Autodesk Inventor part; units mm, degrees
ref_plane "YZ Plane" through (0, 0, 0) normal (1, 0, 0) x (0, 1, 0)
ref_plane "XZ Plane" through (0, 0, 0) normal (0, 1, 0) x (-1, 0, 0)
ref_plane "XY Plane" through (0, 0, 0) normal (0, 0, 1) x (1, 0, 0)
sketch "スケッチ1" plane through (0, 0, 0) normal (0, 0, 1) x (1, 0, 0)
  circle A0 centre (0, 0) radius 2.5
  dimension "d0" = 5
extrude "押し出し1" add sketch "スケッチ1" along normal blind 7.7
fillet "フィレット1" radius 2.5 1 edges at (-2.5, 0, 7.7)
sketch "スケッチ2" plane through (0, 0, 0) normal (0, 0, -1) x (-1, 0, 0)
  circle A0 centre (0, 0) radius 2.9
  line L0 (2.5, 1.4697) -> (2.5, -1.4697)
  circle A1 centre (0, 0) radius 2.5
  dimension "d4" = 5.8
extrude "押し出し2" add sketch "スケッチ2" along normal blind 1 contours A1 | L0 A0 picked at (2.1443, -1.7224)
sketch "スケッチ3" plane through (0, 0, -1) normal (0, 0, -1) x (-1, 0, 0)
  line L0 (-1.52, 0.25) -> (-1.02, 0.25)
  line L1 (-1.02, 0.25) -> (-1.02, -0.25)
  line L2 (-1.02, -0.25) -> (-1.52, -0.25)
  line L3 (-1.52, -0.25) -> (-1.52, 0.25)
  line L4 (1.02, 0.25) -> (1.52, 0.25)
  line L5 (1.52, 0.25) -> (1.52, -0.25)
  line L6 (1.52, -0.25) -> (1.02, -0.25)
  line L7 (1.02, -0.25) -> (1.02, 0.25)
  line L8 (0, 1.603) -> (0, -1.603) construction
  line L9 (-1.27, -1.601) -> (-1.27, 1.6049) construction
  line L10 (1.27, 1.6049) -> (1.27, -1.601) construction
  point P0 (0, 0)
  point P1 (-1.02, 0)
  point P2 (1.02, 0)
  point P3 (0, 0)
  point P4 (-1.27, 0.25)
  point P5 (1.27, 0.25)
  dimension "d7" = 0.5
  dimension "d8" = 0.5
  dimension "d9" = 2.54
extrude "押し出し3" add sketch "スケッチ3" along normal blind 5
properties part number "LED"
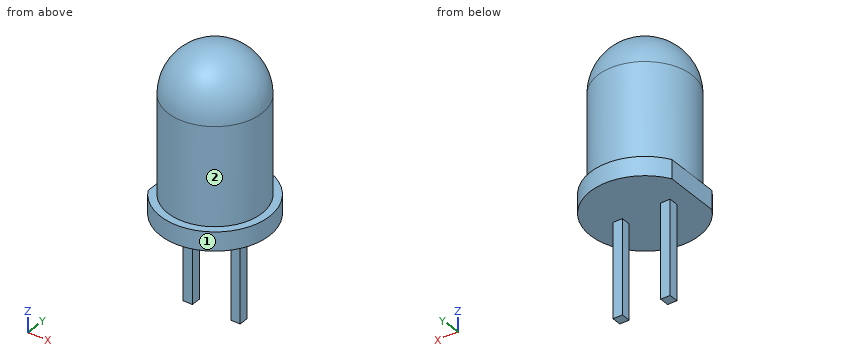
Geometry: final body of the model. Coordinates: model frame, mm. Face numbers are marked on the shaded views. A direction names the side the tool comes from. Give positions to 0.01 mm unless a question says otherwise; leave off trailing zeros. Write each loop counter-clockwise with the first axis right and the second up, starting at its lowest first coordinate (ties: lowest second). Pieces come first, ordered by that corner, then holes.
(1) Cut plane A-A, the plane z = -1.5. Return loops of the section in (x, y).
(2) Cut plane B-B, the plane x = 0. Return loops of the section in (y, z).
(3) Cut plane C-C, the plane y = -0.45. Return loops of the section in (x, z).
(4) Ray query, line 1 (X direction, y = 0.05, z = -4); line 2 (Y direction, x = -1.15, z = -2); line 3 (Z direction, x = 1.6, y = -2.3). Return the intervals inside material, ascending.
(5) First-contact query: P1, Ø2, axis at x = -1, y = -0.5, coming from the +Z side; P2, Ø1.6, axis at x = 1, y = 0, coming from the -Z side; P3, Ø0.6, axis at x = -1.5, z = -4.5, coming from the -Y side. Flat tips, straight axial feed; report the tip coordinate or a pass-through.
(6) Cut plane D-D, the plane z = 5. Return loops of the section in (x, y), then the cut area to 3 significant figures.
(7) Access query for the marked faces 1 and 2. Directions: +Z, -Z, +X, -X, +Y, -Y. A direction counts if a zero-diameter tool reaches every point of the face in a straight line with its end or side. Return the directions, or none.
Values follow:
1. outline: (-1.52, -0.25) - (-1.02, -0.25) - (-1.02, 0.25) - (-1.52, 0.25) - close; (1.02, -0.25) - (1.52, -0.25) - (1.52, 0.25) - (1.02, 0.25) - close
2. outline: (-2.9, -1) - (2.9, -1) - (2.9, 0) - (2.5, 0) - (2.5, 5.2) arc R2.5 ccw to (-2.5, 5.2) - (-2.5, 0) - (-2.9, 0) - close
3. outline: (-2.5, -1) - (2.86, -1) - (2.86, 0) - (2.46, 0) - (2.46, 5.2) arc R2.46 ccw to (-2.46, 5.2) - (-2.46, 0) - (-2.5, 0) - close
4. line 1: x = -1.52 to -1.02, 1.02 to 1.52
4. line 2: y = -0.25 to 0.25
4. line 3: z = -1 to 0
5. P1: stops at z = 7.7
5. P2: stops at z = -6
5. P3: stops at y = -0.25
6. outline: circle Ø5 at (0, 0)
6. area: 19.6 mm2
7. face 1: +Z, -Z
7. face 2: +Z
